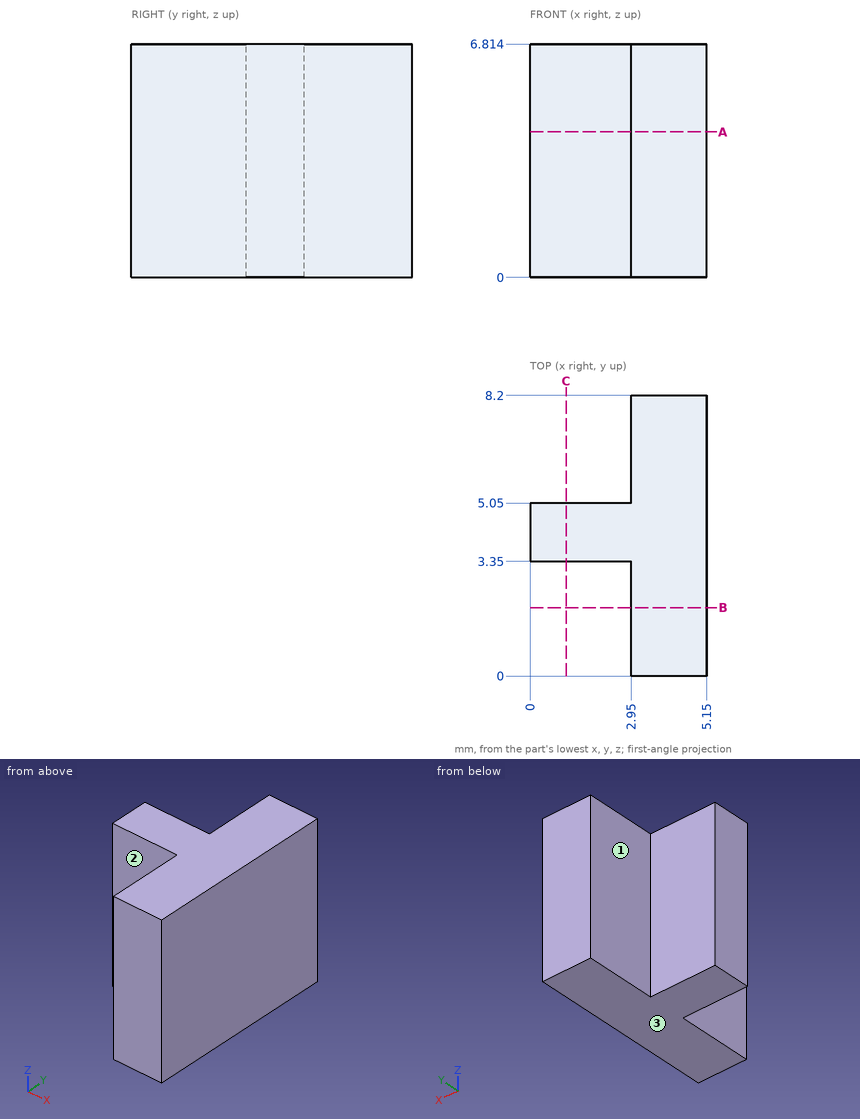
Job drawing, mm, ordinate dimensions from the low corner. One solid piece. A direction names the side the tool comes from. Round coordinates to 2 decimals unless told otherwise and drop trailing zeros. Loops run counter-clockwise (first coordinate to the right, second up) from the corner with the lowest first, then second, coordinate; pieces in that order, holes last. Notation, with made-up numbers: (-23, 57) -> (7, 57) arc R16 ccw to (7, 77) -> close; hole circle Ø6 at (87.5, 65.25). An arc over 180 degrees is marked (long way). Use CSV: the item, a comma, the result in double quotes. Start each with the question number.
Q1. Flat gauge pins, fed straight in: pin 1 Ø1.6 at (y, z) = (7, 4) entering from -X; pin 2 Ø3 at (y, z) = (2, 3) entering from -X. Where does each tip first touch, or does it go through?
Q2. Saw through at B-B on y = 2. Give the cut face in (x, z), and give its area (3 significant figures).
Q3. Saw through at A-A on z = 4.25. Give the cut face in (x, y), and give its area (3 significant figures).
Q4. Which spindle directions (+Z, -Z, +X, -X, +Y, -Y) get a long thin tool onto all of the face, cutting with end or side? Do the marked faces 1, 2 and 3. Say none if no direction does.
Q5. Drill centre lines: L1, parallel to Y at x = 1.7, z = 5.5; L2, parallel to X at y = 0.75, z = 2.5. Where is each one in solid material? Low to high.
Q6. Saw through at C-C on x = 1.05. Give the cut face in (y, z), and give its area (3 significant figures).
Solutions:
1,pin 1,"stops at x = 2.95"
1,pin 2,"stops at x = 0"
2,outline,"(2.95, 0) -> (5.15, 0) -> (5.15, 6.81) -> (2.95, 6.81) -> close"
2,area,"15.0 mm^2"
3,outline,"(0, 3.35) -> (2.95, 3.35) -> (2.95, 0) -> (5.15, 0) -> (5.15, 8.2) -> (2.95, 8.2) -> (2.95, 5.05) -> (0, 5.05) -> close"
3,area,"23.1 mm^2"
4,face 1,"+Z, -Z, -X, +Y"
4,face 2,"+Z, -Z, -X, -Y"
4,face 3,"-Z, +X, -X, +Y, -Y"
5,L1,"y = 3.35 to 5.05"
5,L2,"x = 2.95 to 5.15"
6,outline,"(3.35, 0) -> (5.05, 0) -> (5.05, 6.81) -> (3.35, 6.81) -> close"
6,area,"11.6 mm^2"
